Part print with two shaded views. Sizes in mm from the minimum x, y, z corner. A direction names the side the tool comes from. Round coordinates to 2 decimals unless told otherwise and drop trailing zeros. Order: outer loops, then holes, each group sorted by start corner. A loop starts at its lowest first (then second) coordinate and runs counter-clockwise, first axis right, second up. Notation, with made-up numbers: M 89,72.5 L 124,72.5 A20 cw 124,91.5 Z; hole C -11.75,-25 d9. An arc over 180 degrees is marked long. Answer as a JSON object with one key per item and string values.
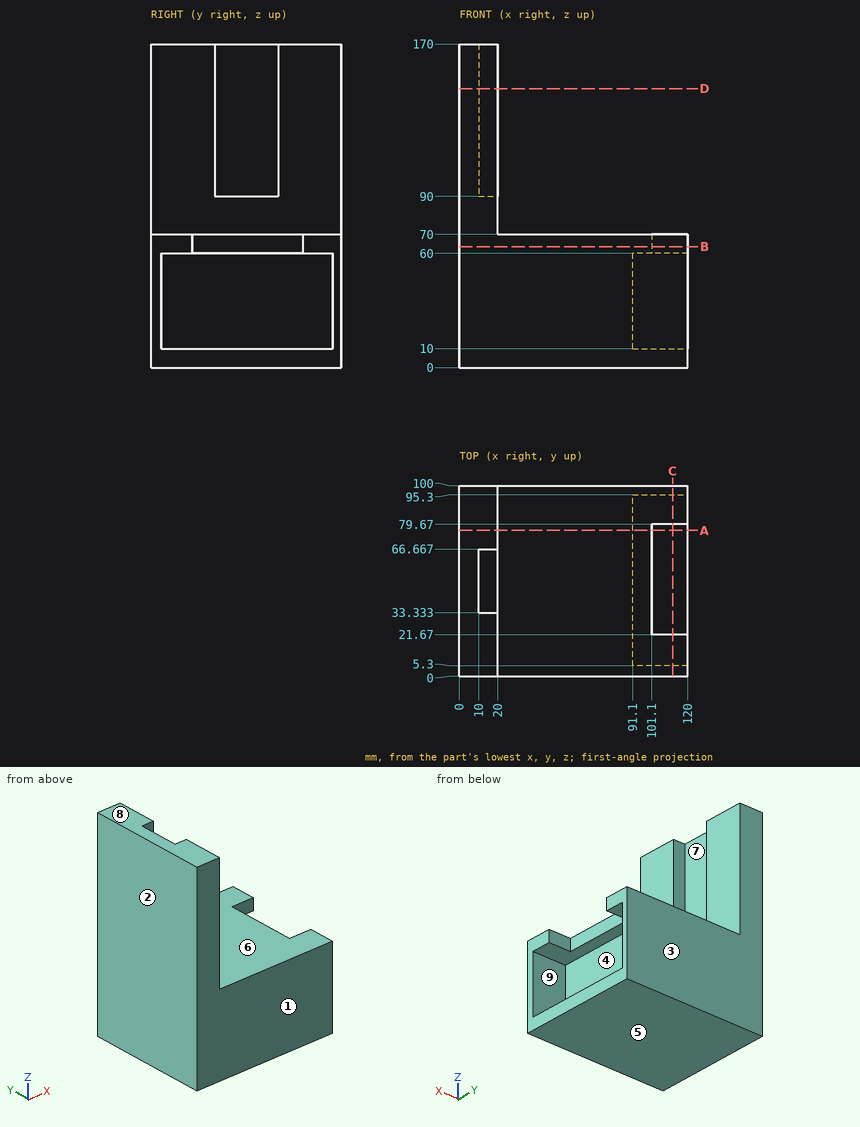
Item 1: Saw through at C-C on x = 112. List the corners of the cut face in (y, z).
Worked answers:
{"outline": "M 0,0 L 100,0 L 100,70 L 79.67,70 L 79.67,60 L 95.3,60 L 95.3,10 L 5.3,10 L 5.3,60 L 21.67,60 L 21.67,70 L 0,70 Z"}
Item 2: Two-plate mould, pull along Y, no slides. Class the marked faces 1, 2, 3 and 4: released by +Y, released by -Y, zero draft, split by the parting line, or undercut.
Worked answers:
{"face 1": "released by -Y", "face 2": "zero draft", "face 3": "released by +Y", "face 4": "undercut"}
Item 3: Saw through at D-D on z = 146.5. List the corners of the cut face in (x, y).
Worked answers:
{"outline": "M 0,0 L 20,0 L 20,33.33 L 10,33.33 L 10,66.67 L 20,66.67 L 20,100 L 0,100 Z"}
Item 4: 3-axis set-ups, long thin cutter, end or side, ignore diameter. For the marked faces 5, 6, 7, 8 and 9: which of +Z, -Z, +X, -X, +Y, -Y reach the whole face in a straight line?
Worked answers:
{"face 5": "-Z, +X, -X, +Y, -Y", "face 6": "+Z, +X, +Y, -Y", "face 7": "+Z, +X", "face 8": "+Z, +X, -X, +Y, -Y", "face 9": "+X"}
Item 5: Wall check: line 1 along Z through (x, y) = (101, 23); line 2 along Z through (x, y) = (76, 34); line 3 along X through (y, z) = (56, 10.5). Give the ranges that are in metal, low to high. Write a range as [from, to].
Worked answers:
{"line 1": "z = [0, 10], [60, 70]", "line 2": "z = [0, 70]", "line 3": "x = [0, 91.1]"}
Item 6: Saw through at B-B on z = 63.5. List the corners of the cut face in (x, y).
Worked answers:
{"outline": "M 0,0 L 120,0 L 120,21.67 L 101.1,21.67 L 101.1,79.67 L 120,79.67 L 120,100 L 0,100 Z"}
Item 7: Saw through at A-A on y = 76.5. List the corners of the cut face in (x, z), and give its area (3 significant figures).
Worked answers:
{"outline": "M 0,0 L 120,0 L 120,10 L 91.1,10 L 91.1,60 L 101.1,60 L 101.1,70 L 20,70 L 20,170 L 0,170 Z", "area": "8,770 mm2"}
Item 8: Drop flat-ended pins along their axis: pin 1 Ø1 at (y, z) = (80, 27) entering from +X; pin 2 Ø11 at (y, z) = (51.5, 65) entering from +X; pin 3 Ø8 at (x, y) = (16.5, 51.5) entering from +Z. Give the stop position or say it passes through.
Worked answers:
{"pin 1": "stops at x = 91.1", "pin 2": "stops at x = 101.1", "pin 3": "stops at z = 90"}
